from build123d import *

# Parameters (mm, degrees)
SKETCH_1_W           = 2.54
SKETCH_1_H           = 6.2
EXTRUDE_1_DEPTH      = 3
SKETCH_2_W           = 1.2
SKETCH_2_H           = 2
CUT_EXTRUDE_1_DEPTH  = 0.5
SKETCH_3_W           = 1
SKETCH_3_H           = 1
EXTRUDE_1_2_DEPTH    = 1
FILLET_1_R           = 0.3
CHAMFER_1_SIZE       = 0.4
CHAMFER_1_SIZE2      = 1.098990968
EXTRUDE_2_DEPTH      = 0.45
EXTRUDE_2_DEPTH_BACK = 0.45
SKETCH_5_W           = 0.25
SKETCH_5_H           = 0.807139358
CUT_EXTRUDE_2_DEPTH  = 0.45


with BuildPart() as part:
    # 草图1 → Extrude 1 (new body)
    with BuildSketch(Plane(origin=(0, 0, 0), x_dir=(1, 0, 0), z_dir=(0, 1, 0))):
        Rectangle(SKETCH_1_W, SKETCH_1_H)
    extrude(amount=EXTRUDE_1_DEPTH)

    # 草图2 → 切除-拉伸1 (cut)
    with BuildSketch(Plane(origin=(0, 3, 0), x_dir=(1, 0, 0), z_dir=(0, 1, 0))):
        Rectangle(SKETCH_2_W, SKETCH_2_H)
    extrude(amount=-CUT_EXTRUDE_1_DEPTH, mode=Mode.SUBTRACT)

    # 草图3 → Extrude 1 2 (add)
    with BuildSketch(Plane(origin=(0, 2.5, 0), x_dir=(1, 0, 0), z_dir=(0, 1, 0))):
        with Locations((0, 0.4)):
            Rectangle(SKETCH_3_W, SKETCH_3_H)
    extrude(amount=EXTRUDE_1_2_DEPTH)

    # 圆角1
    fillet_1_edges = [part.edges().sort_by_distance(p)[0] for p in [
        (0, 3, -3.1),
        (0, 3, 3.1),
    ]]
    fillet(fillet_1_edges, radius=FILLET_1_R)

    # 倒角1
    chamfer_1_edges = [part.edges().sort_by_distance(p)[0] for p in [
        (0, 0, -3.1),
        (0, 0, 3.1),
    ]]
    chamfer_1_side = [part.faces().sort_by_distance(p)[0] for p in [
        (0, 0, 0),
    ]]
    chamfer(chamfer_1_edges, length=CHAMFER_1_SIZE, length2=CHAMFER_1_SIZE2, reference=chamfer_1_side[0])

    # 草图4 → 凸台-拉伸2 (add, two sides: drawn at the far end of the back side and taken through both)
    with BuildSketch(Plane(origin=(0, 0, 0), x_dir=(0, 0, -1), z_dir=(1, 0, 0)).offset(-EXTRUDE_2_DEPTH_BACK)):
        Polygon((-2.942106966, 1.594783958), (-3.595340284, 1.594783958), (-3.89950168, -0.245392483), (-4.9, -0.245392483), (-4.9, -0.445392483), (-3.729845887, -0.445392483), (-3.425684492, 1.394783958), (-2.942106966, 1.394783958), align=None)
        Polygon((2.942106966, 1.394783958), (2.942106966, 1.594783958), (3.595340284, 1.594783958), (3.89950168, -0.245392483), (4.9, -0.245392483), (4.9, -0.445392483), (3.729845887, -0.445392483), (3.425684492, 1.394783958), align=None)
    extrude(amount=EXTRUDE_2_DEPTH + EXTRUDE_2_DEPTH_BACK)

    # 草图5 → 切除-拉伸2 (cut)
    with BuildSketch(Plane(origin=(0, -0.245392483, 0), x_dir=(1, 0, 0), z_dir=(0, 1, 0))):
        with Locations((0.325, 4.496430321)):
            Rectangle(SKETCH_5_W, SKETCH_5_H)
        with Locations((-0.325, 4.496430321)):
            Rectangle(SKETCH_5_W, SKETCH_5_H)
        with Locations((0.325, -4.496430321)):
            Rectangle(SKETCH_5_W, SKETCH_5_H)
        with Locations((-0.325, -4.496430321)):
            Rectangle(SKETCH_5_W, SKETCH_5_H)
    extrude(amount=-CUT_EXTRUDE_2_DEPTH, mode=Mode.SUBTRACT)


solid = part.part
Here's how the part is built. I have some questions about the finished solid (model axes, mm). A direction names the side the tool comes from. Round coordinates to 2 decimals unless told otherwise and drop trailing zeros. Order: outer loops, then holes, each group sorted by start corner. A loop starts at its lowest first (then second) coordinate and runs counter-clockwise, first axis right, second up. Notation, with made-up numbers: (81.5, 51.5) -> (112.5, 51.5) arc R25 ccw to (112.5, 79.5) -> close; hole circle Ø2 at (35, 27). An arc over 180 degrees is marked (long way). Use CSV: the item, a comma, the result in double quotes.
1. I want a section at A-A on y = 0.4. List the corners of the cut face in (x, z) for me, and give its area (3 significant figures).
Recorded:
outline,"(-1.27, -2.85) -> (1.27, -2.85) -> (1.27, 2.85) -> (-1.27, 2.85) -> close; (-0.45, -3.79) -> (0.45, -3.79) -> (0.45, -3.59) -> (-0.45, -3.59) -> close; (-0.45, 3.59) -> (0.45, 3.59) -> (0.45, 3.79) -> (-0.45, 3.79) -> close"
area,"14.8 mm2"
2. Thinking about a two-plate mould opening in Z: for faces 6 (the face through (-0.006, 0.688, 3.745)), 7 (the face through (0, 2.5, 0.4)), 8 (the face through (0, -0.445, 4)), 9 (the face through (-0.01, 0.46, -3.58)), which applies, pulls with the +Z half, pulls with the -Z half, needs draft (parallel to the pull), parting line crosses it, or undercut?
Recorded:
face 6,"pulls with the +Z half"
face 7,"undercut"
face 8,"needs draft"
face 9,"undercut"
3. I want a section at D-D on y = 1.9. List the corners of the cut face in (x, z) for me.
Recorded:
outline,"(-1.27, -3.1) -> (1.27, -3.1) -> (1.27, 3.1) -> (-1.27, 3.1) -> close"
4. I want a section at B-B on z = 0.5. List the corners of the cut face in (x, y) for me.
Recorded:
outline,"(-1.27, 0) -> (1.27, 0) -> (1.27, 3) -> (0.6, 3) -> (0.6, 2.5) -> (-0.6, 2.5) -> (-0.6, 3) -> (-1.27, 3) -> close"
5. I'm going to push flat-ended pins straight in: P1, Ø1.3, axis at x = 0.5, y = 2, coming from the -Z side; P2, Ø0.5, axis at x = 0, z = 3.5, coming from the +Y side; P3, Ø0.5, axis at x = -0.5, y = 2, coming from the +Z side. Where does each tip first touch, or does it pass through?
Recorded:
P1,"stops at z = -3.64"
P2,"stops at y = 1.59"
P3,"stops at z = 3.1"
6. I need wall thicknesses on line 1 along X through (y, z) = (-0.15, 3.75); line 2 along Y through (x, z) = (0.05, 0.25); line 3 along Y through (x, z) = (-0.55, 2). Which ranges of each line are inside material? Lowest first, please.
Recorded:
line 1,"x = -0.45 to 0.45"
line 2,"y = 0 to 2.5"
line 3,"y = 0 to 3"
7. Which directions (+Z, -Z, +X, -X, +Y, -Y) give clear straight access to the entire face, cutting with the end or side of a thin tool? Please do faces 1 (the face through (-0.018, 0.557, -2.903)), 2 (the face through (0, 3, 0.1)), 3 (the face through (0, -0.245, 4.3)), 4 (the face through (0, -0.445, -4)), 5 (the face through (0, -0.245, -4.3)).
Recorded:
face 1,"+X, -X, -Y"
face 2,"+Y"
face 3,"+Z, +X, -X, +Y"
face 4,"+Z, -Z, +X, -X, -Y"
face 5,"-Z, +X, -X, +Y"
